Design review of the part built by this model. Coordinates are the model's own, in mm. Face numbers are marked on the shaded views. A direction names the side the tool comes from. Give positions to 0.01 mm unless a question says otherwise; leave off trailing zeros. Loops run counter-clockwise (first coordinate to the right, second up) from the corner with the lowest first, then second, coordinate; pieces in that order, holes last. Notation, with made-up numbers: (59, 35) -> (68, 35) arc R13 cw to (68, 45) -> close; hole circle Ø2 at (-12, 18). An arc over 180 degrees is marked (long way). Use CSV: the item, a comma, the result in double quotes. Start each with the question number.
Item 1: We need section C-C (z = 3.5). State the section outline as (x, y) points.
Item 2: We need section A-A (y = 0). State the section outline as (x, z) points.
Item 3: Wall thickness on line 1 along Z through (x, y) = (14, 0); line 2 along Y through (x, z) = (0, 5); line 3 along Y through (x, z) = (8.5, 1.25): over which ranges is each line inside the solid? List them lowest first. Write a range as from..to.
Item 4: We need section B-B (x = 0). State the section outline as (y, z) points.
Item 5: Clearance check with a flat-ended pin moving along its axis: pin 1 (3 mm diameter, centred on x = -8, z = 5, fed in from +Y). State where the tip first meets the part, or that it passes through.
Item 6: For the marked faces 4, 5 and 6, list the 3-axis set-ups (+Z, -Z, +X, -X, +Y, -Y) from which the entire face can be reached by the end or side of a thin tool; tool diameter is ignored.
Item 7: We need section D-D (z = 1). State the section outline as (x, y) points, plus the area to 3 significant figures.
Item 8: The part is to be moulded in two halves that separate along X. For the marked faces 1, 2 and 3, say which applies: +X half, -X half, draft (parallel to the pull), parting line (faces both ways), or undercut.
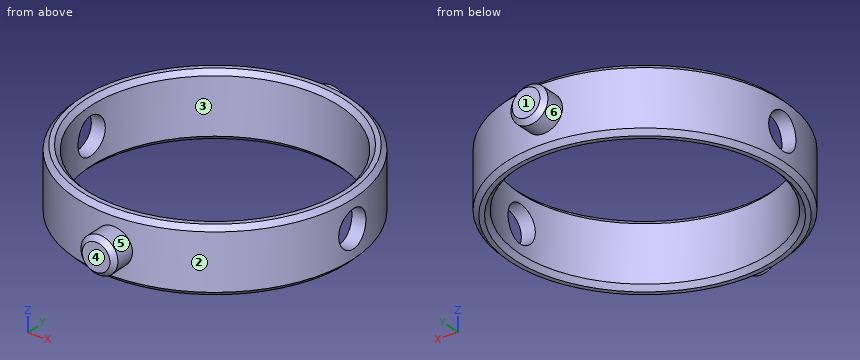
from build123d import *

# Parameters (mm, degrees)
F0_R     = 15
F0_R_2   = 13.5
F1_DEPTH = 7
F2_R     = 2
F3_DEPTH = 20
F4_SIZE  = 0.5
F6_R     = 2
F7_DEPTH = 4
F9_SIZE  = 0.5


with BuildPart() as f1:
    # F0 (on Top) → F1 (new body)
    with BuildSketch(Plane.XY):
        Circle(F0_R)
        Circle(F0_R_2, mode=Mode.SUBTRACT)
    extrude(amount=F1_DEPTH)

    # F2 (on Right) → F3 (cut, symmetric)
    with BuildSketch(Plane.YZ):
        with Locations((0, 3.5)):
            Circle(F2_R)
    extrude(amount=F3_DEPTH, both=True, mode=Mode.SUBTRACT)

    # F4
    f4_edges = [f1.edges().sort_by_distance(p)[0] for p in [
        (-15, 0, 7),
        (-13.5, 0, 7),
        (-15, 0, 0),
        (-13.5, 0, 0),
    ]]
    chamfer(f4_edges, length=F4_SIZE)

    # F6 (on offset) → F7 (join)
    with BuildSketch(Plane.XZ.offset(-13.5)):
        with Locations((0, 3.5)):
            Circle(F6_R)
    extrude(amount=-F7_DEPTH)

    # F8: F1 across plane


with BuildPart() as f1_1:
    add(f1.part)
    add(f1.part.mirror(Plane.XZ))

    # F9
    f9_edges = [f1_1.edges().sort_by_distance(p)[0] for p in [
        (-2, 17.5, 3.5),
        (-2, -17.5, 3.5),
    ]]
    chamfer(f9_edges, length=F9_SIZE)


solid = f1_1.part
Results found:
1,outline,"(-14.87, -2) arc R15 ccw to (-2, -14.87) -> (-2, -17) -> (-1.5, -17.5) -> (1.5, -17.5) -> (2, -17) -> (2, -14.87) arc R15 ccw to (14.87, -2) -> (13.35, -2) arc R13.5 cw to (-13.35, -2) -> close; (-14.87, 2) -> (-13.35, 2) arc R13.5 cw to (13.35, 2) -> (14.87, 2) arc R15 ccw to (2, 14.87) -> (2, 17) -> (1.5, 17.5) -> (-1.5, 17.5) -> (-2, 17) -> (-2, 14.87) arc R15 ccw to start"
2,outline,"(-15, 0.5) -> (-14.5, 0) -> (-14, 0) -> (-13.5, 0.5) -> (-13.5, 1.5) -> (-15, 1.5) -> close; (-15, 5.5) -> (-13.5, 5.5) -> (-13.5, 6.5) -> (-14, 7) -> (-14.5, 7) -> (-15, 6.5) -> close; (13.5, 0.5) -> (14, 0) -> (14.5, 0) -> (15, 0.5) -> (15, 1.5) -> (13.5, 1.5) -> close; (13.5, 5.5) -> (15, 5.5) -> (15, 6.5) -> (14.5, 7) -> (14, 7) -> (13.5, 6.5) -> close"
3,line 1,"0..1.5, 5.5..7"
3,line 2,"-17.5..-13.5, 13.5..17.5"
3,line 3,"-12.36..-10.49, 10.49..12.36"
4,outline,"(-17.5, 2) -> (-17, 1.5) -> (-15, 1.5) -> (-15, 0.5) -> (-14.5, 0) -> (-14, 0) -> (-13.5, 0.5) -> (-13.5, 6.5) -> (-14, 7) -> (-14.5, 7) -> (-15, 6.5) -> (-15, 5.5) -> (-17, 5.5) -> (-17.5, 5) -> close; (13.5, 0.5) -> (14, 0) -> (14.5, 0) -> (15, 0.5) -> (15, 1.5) -> (17, 1.5) -> (17.5, 2) -> (17.5, 5) -> (17, 5.5) -> (15, 5.5) -> (15, 6.5) -> (14.5, 7) -> (14, 7) -> (13.5, 6.5) -> close"
5,pin 1,"y = 13.52"
6,face 4,"+Z, -Z, +X, -X, -Y"
6,face 5,"-Y"
6,face 6,"+Y"
7,outline,"circle Ø30 at (0, 0); hole circle Ø27 at (0, 0)"
7,area,"134 mm²"
8,face 1,"draft"
8,face 2,"parting line"
8,face 3,"undercut"
